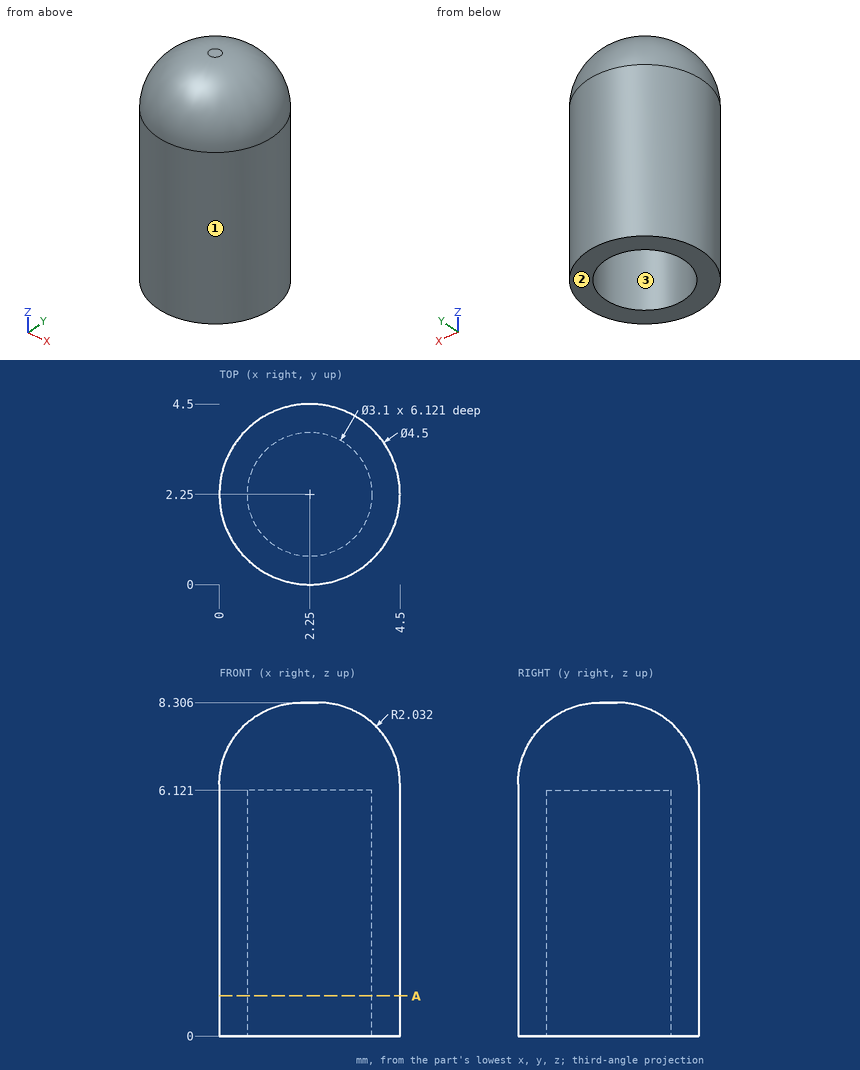
The drawing under review shows one solid part. Ordinate dimensions are in mm from its lowest x, y, z. Round coordinates to 2 decimals unless told otherwise and drop trailing zeros. Write each loop counter-clockwise with the first axis right and the second up, starting at its lowest first coordinate (ties: lowest second). Pieces come first, ordered by that corner, then holes. Notation, with made-up numbers: M 19.25,36.5 L 65.25,36.5 A20 cw 65.25,55.5 Z; hole C 44,4.5 d3. An arc over 180 degrees is marked long. One line per item, written item: value. Start each with the question number.
(1) The part is to be moulded in two halves that separate along Y. For the marked faces 1, 2 and 3, say which applies: released by +Y, released by -Y, zero draft, split by the parting line, or undercut.
(2) We need section A-A (z = 1). Give the boundary of the cut face in (x, y).
(3) Insertion check: pin 1 (2 mm diameter, centred on x = 2.5, y = 4, fed in from +Z); pin 2 (2.5 mm diameter, centred on x = 2.25, y = 2.25, fed in from -Z). Each pin has a flat end and moves straight along its axis. Give the tip position at first contact, or say it passes through.
(4) Wall thickness on line 1 (Y direction, x = 2.25, z = 4.25); line 2 (Y direction, x = 2.75, z = 1.75) (1 decimal); line 3 (X direction, y = 2.7, z = 7.25): over which ranges is each line inside the solid? List them lowest first.
Result:
1. face 1: split by the parting line
1. face 2: zero draft
1. face 3: undercut
2. outline: C 2.25,2.25 d4.5; hole C 2.25,2.25 d3.1
3. pin 1: z = 8.23
3. pin 2: z = 6.12
4. line 1: 0 to 0.7, 3.8 to 4.5
4. line 2: 0.1 to 0.8, 3.7 to 4.4
4. line 3: 0.3 to 4.2
